Source: CAD feature listing. Evaluate the final solid. Frame: model axes, mm. A direction names the side the tool comes from. Round coordinates to 2 decimals unless told otherwise and drop trailing zeros. Loops run counter-clockwise (first coordinate to the right, second up) from the corner with the lowest first, then second, coordinate; pieces in that order, holes last. Notation, with made-up numbers: M -1,-17 L 15,-17 A22 ccw 15,16 Z; hole C 61.5,50 d7. An arc over 180 degrees is marked long. Write each question's results on one line, items separated by ' | '. Start each with the question number.
1. Set-up query: faces 1 (the flat face through (-79.23, 22.07, 17.185)), 2 (the flat face through (-25, 47, -22)), 3 (the flat face through (-2, 0, -1)). Return all of +Z, -Z, +X, -X, +Y, -Y with unobstructed straight access to the full face (end or side cutting, diameter ignored); none if empty.
2. Section C-C on x = -7.5. Output: boundary loops of the cut face in (y, z), and give its area (3 significant figures).
3. Contact query for flat-ended pins moving along their axis: pin 1 Ø4 at (x, y) = (-56.5, 65.5) entering from +Z; pin 2 Ø2 at (x, z) = (25.5, 30) entering from +Y; pin 3 Ø17.5 at (x, z) = (-3.5, -14) entering from +Y. Output: stop coordinate, or through.
4. Section B-B on z = -30. Output: boundary loops of the cut face in (x, y).
5. Section A-A on y = 21.5. Output: boundary loops of the cut face in (x, z).
6. Ray query, line 1 (X direction, y = 56.5, z = -11); line 2 (X direction, y = 33.5, z = 16.5); line 3 (Y direction, x = -110.5, z = 14). Return the intervals inside material, ascending.
7. Section D-D on y = 41.5. Output: boundary loops of the cut face in (x, z), and give its area (3 significant figures).
8. Draft query along X for faces 4 (the flat face through (-135, 31, -8)), 5 (the flat face through (0, 14.403, -22)), 6 (the flat face through (-81, 80, -23)). Return one class per face: released by +X, released by -X, zero draft, split by the parting line, or undercut.
from build123d import *

# Parameters (mm, degrees)
SKETCH1_W           = 270
SKETCH1_H           = 80
BOSS_EXTRUDE1_DEPTH = 80
CUT_EXTRUDE1_DEPTH  = 81
BOSS_EXTRUDE2_DEPTH = 270
SKETCH3_R           = 45
CUT_EXTRUDE2_DEPTH  = 271
SKETCH5_W           = 50
SKETCH5_H           = 65.597147321
CUT_EXTRUDE3_DEPTH  = 36


with BuildPart() as part:
    # Sketch1 → Boss-Extrude1 (new body)
    with BuildSketch(Plane(origin=(0, 0, 0), x_dir=(1, 0, 0), z_dir=(0, 1, 0))):
        Rectangle(SKETCH1_W, SKETCH1_H)
    extrude(amount=BOSS_EXTRUDE1_DEPTH)

    # Sketch2 → Cut-Extrude1 (cut, through all)
    with BuildSketch(Plane(origin=(0, 80, 0), x_dir=(1, 0, 0), z_dir=(0, 1, 0))):
        Polygon((0, -40), (0, 5), (-25, 5), (-135, -40), align=None)
        Polygon((135, -40), (25, 5), (0, 5), (0, -40), align=None)
    extrude(amount=-CUT_EXTRUDE1_DEPTH, mode=Mode.SUBTRACT)

    # Sketch4 → Boss-Extrude2 (add)
    with BuildSketch(Plane(origin=(135, 0, 0), x_dir=(0, 0, -1), z_dir=(1, 0, 0))):
        with BuildLine():
            Line((40, 80), (37.459666924, 80))
            ThreePointArc((37.459666924, 80), (15.677643628, 23.590353368), (-40, 0))
            Line((-40, 0), (40, 0))
            Line((40, 0), (40, 80))
        make_face()
    extrude(amount=-BOSS_EXTRUDE2_DEPTH)

    # Sketch3 → Cut-Extrude2 (cut, through all)
    with BuildSketch(Plane(origin=(135, 0, 0), x_dir=(0, 0, -1), z_dir=(1, 0, 0))):
        with Locations((-40, 77.5)):
            Circle(SKETCH3_R)
    extrude(amount=-CUT_EXTRUDE2_DEPTH, mode=Mode.SUBTRACT)

    # Sketch5 → Cut-Extrude3 (cut, through all)
    with BuildSketch(Plane.XY.offset(-5)):
        with Locations((0, 47.20142634)):
            Rectangle(SKETCH5_W, SKETCH5_H)
    extrude(amount=-CUT_EXTRUDE3_DEPTH, mode=Mode.SUBTRACT)


solid = part.part
Taken from the geometry:
1) face 1: +Z, +Y | face 2: +Z, -Z, +Y | face 3: +Z, -Z, +X, -X, -Y
2) outline: M 0,-40 L 14.4,-40 L 14.4,-5 A77.5 cw 0,40 Z | area: 711 mm^2
3) pin 1: z = -2.77 | pin 2: y = 0.78 | pin 3: y = 14.4
4) outline: M -135,0 L 135,0 L 135,80 L 25,80 L 25,14.4 L -25,14.4 L -25,80 L -135,80 Z
5) outline: M -135,-40 L -25,-40 L -25,-5 L -135,40 Z; M 25,-40 L 135,-40 L 135,40 L 25,-5 Z
6) line 1: -135 to -25, 25 to 135 | line 2: -135 to -77.56, 77.56 to 135 | line 3: 0 to 40.77
7) outline: M -135,-40 L -25,-40 L -25,-5 L -69,13 L -135,13 Z; M 25,-40 L 135,-40 L 135,13 L 69,13 L 25,-5 Z | area: 10,900 mm^2
8) face 4: released by -X | face 5: undercut | face 6: zero draft
